Read the model definition and answer for the solid it produces. Units are mm, in the model's axes. Face numbers are marked on the shaded views. A direction names the side the tool comes from. Give positions to 0.01 mm unless a question says otherwise; leave off trailing zeros. Order: outer loops, then holes, each group sorted by start corner. A loop starts at its lowest first (then second) coordinate and runs counter-clockwise, first axis right, second up. Notation, with made-up numbers: (3.5, 81) -> (22.5, 81) arc R22 cw to (22.5, 111) -> close; hole circle Ø6 at (32, 8). An arc over 180 degrees is marked (long way). Use one line per item in the form item = value.
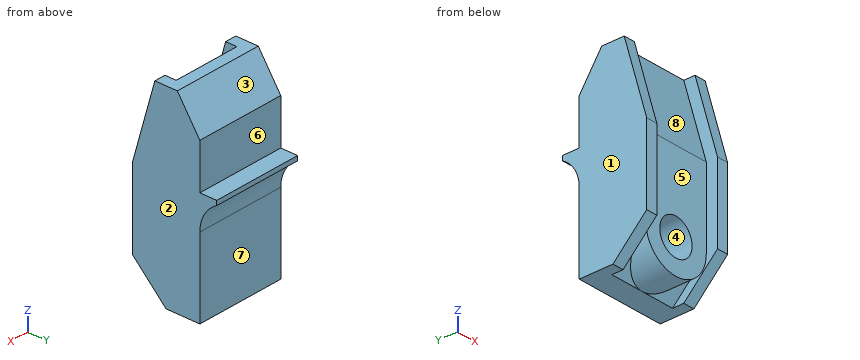
```python
from build123d import *

# Parameters (mm, degrees)
CYLINDER460_R     = 1.6
CYLINDER460_DEPTH = 10
CYLINDER461_R     = 3
CYLINDER461_DEPTH = 3
BOX316_W          = 8
BOX316_H          = 7.5
BOX316_DEPTH      = 17
CHAMFER036_SIZE   = 3
CHAMFER037_SIZE2  = 2
CHAMFER037_SIZE   = 7
BOX317_W          = 6
BOX317_H          = 7.5
BOX317_DEPTH      = 17
BOX314_W          = 10
BOX314_H          = 3
BOX314_DEPTH      = 12
BOX313_W          = 10
BOX313_H          = 3
BOX313_DEPTH      = 12
FILLET112_R       = 2.99
BOX312_W          = 8
BOX312_H          = 7.5
BOX312_DEPTH      = 17
CHAMFER033_SIZE   = 3
CHAMFER034_SIZE2  = 2
CHAMFER034_SIZE   = 7
CHAMFER035_SIZE2  = 3
CHAMFER035_SIZE   = 2


with BuildPart() as cylinder574:
    # Cylinder460 → Cylinder460 (new body)
    with BuildSketch(Plane(origin=(120, -21, 13), x_dir=(1, 0, 0), z_dir=(0, 1, 0))):
        Circle(CYLINDER460_R)
    extrude(amount=CYLINDER460_DEPTH)


with BuildPart() as cylinder575:
    # Cylinder461 → Cylinder461 (new body)
    with BuildSketch(Plane(origin=(120, -15, 13), x_dir=(1, 0, 0), z_dir=(0, 1, 0))):
        Circle(CYLINDER461_R)
    extrude(amount=CYLINDER461_DEPTH)


with BuildPart() as chamfer037:
    # Box316 → Box316 (new body)
    with BuildSketch(Plane(origin=(116, -16, 10), x_dir=(1, 0, 0), z_dir=(0, 0, 1))):
        with Locations((4, 3.75)):
            Rectangle(BOX316_W, BOX316_H)
    extrude(amount=BOX316_DEPTH)

    # Chamfer036
    chamfer036_edges = [chamfer037.edges().sort_by_distance(p)[0] for p in [
        (120, -16, 10),
    ]]
    chamfer(chamfer036_edges, length=CHAMFER036_SIZE)

    # Chamfer037
    chamfer037_edges = [chamfer037.edges().sort_by_distance(p)[0] for p in [
        (120, -16, 27),
    ]]
    chamfer037_side = chamfer037.faces().sort_by_distance((120, -16, 20))[0]
    chamfer(chamfer037_edges, length=CHAMFER037_SIZE, length2=CHAMFER037_SIZE2, reference=chamfer037_side)


with BuildPart() as cut312:
    # Box317 → Box317 (new body)
    with BuildSketch(Plane(origin=(117, -20, 10), x_dir=(1, 0, 0), z_dir=(0, 0, 1))):
        with Locations((3, 3.75)):
            Rectangle(BOX317_W, BOX317_H)
    extrude(amount=BOX317_DEPTH)

    # Cut312: cut Chamfer037
    add(chamfer037.part, mode=Mode.SUBTRACT)


with BuildPart() as cut312_1:
    # Cut312 placement: moved
    add(cut312.part.moved(Location((0, 1, 0))))


with BuildPart() as cube385:
    # Box314 → Box314 (new body)
    with BuildSketch(Plane(origin=(116, -10, 20), x_dir=(1, 0, 0), z_dir=(0, 0, 1))):
        with Locations((5, 1.5)):
            Rectangle(BOX314_W, BOX314_H)
    extrude(amount=BOX314_DEPTH)


with BuildPart() as fillet112:
    # Box313 → Box313 (new body)
    with BuildSketch(Plane(origin=(116, -10, 8), x_dir=(1, 0, 0), z_dir=(0, 0, 1))):
        with Locations((5, 1.5)):
            Rectangle(BOX313_W, BOX313_H)
    extrude(amount=BOX313_DEPTH)

    # Fillet112
    fillet112_edges = [fillet112.edges().sort_by_distance(p)[0] for p in [
        (121, -10, 20),
    ]]
    fillet(fillet112_edges, radius=FILLET112_R)


with BuildPart() as kipper_holder_left:
    # Box312 → Box312 (new body)
    with BuildSketch(Plane(origin=(116, -16, 10), x_dir=(1, 0, 0), z_dir=(0, 0, 1))):
        with Locations((4, 3.75)):
            Rectangle(BOX312_W, BOX312_H)
    extrude(amount=BOX312_DEPTH)

    # Chamfer033
    chamfer033_edges = [kipper_holder_left.edges().sort_by_distance(p)[0] for p in [
        (120, -16, 10),
    ]]
    chamfer(chamfer033_edges, length=CHAMFER033_SIZE)

    # Chamfer034
    chamfer034_edges = [kipper_holder_left.edges().sort_by_distance(p)[0] for p in [
        (120, -16, 27),
    ]]
    chamfer034_side = kipper_holder_left.faces().sort_by_distance((120, -16, 20))[0]
    chamfer(chamfer034_edges, length=CHAMFER034_SIZE, length2=CHAMFER034_SIZE2, reference=chamfer034_side)

    # Cut310: cut Fillet112
    add(fillet112.part, mode=Mode.SUBTRACT)

    # Cut311: cut Cube385
    add(cube385.part, mode=Mode.SUBTRACT)

    # Chamfer035
    chamfer035_edges = [kipper_holder_left.edges().sort_by_distance(p)[0] for p in [
        (120, -10, 27),
    ]]
    chamfer035_side = kipper_holder_left.faces().sort_by_distance((120, -12, 27))[0]
    chamfer(chamfer035_edges, length=CHAMFER035_SIZE, length2=CHAMFER035_SIZE2, reference=chamfer035_side)

    # Cut313: cut Cut312
    add(cut312_1.part, mode=Mode.SUBTRACT)

    # Fusion416: union Cylinder575
    add(cylinder575.part)

    # Cut314: cut Cylinder574
    add(cylinder574.part, mode=Mode.SUBTRACT)


solid = kipper_holder_left.part
```
Item 1: The part is cut by section D-D on y = -10.5. Give the vertices of the cut face in (x, z).
Checks:
outline = (116, 10) -> (124, 10) -> (124, 24.75) -> (116, 24.75) -> close
Item 2: The part is cut by section C-C on x = 121. Give the vertices of the cut face in (y, z).
Checks:
outline = (-15, 10.17) -> (-12.17, 10.17) -> (-12, 10) -> (-10, 10) -> (-10, 17.01) arc R2.99 cw to (-8.5, 19.6) -> (-8.5, 20) -> (-10, 20) -> (-10, 24) -> (-12, 27) -> (-13, 27) -> (-15, 20) -> (-15, 14.25) -> (-11, 14.25) -> (-11, 11.75) -> (-15, 11.75) -> close
Item 3: Given pin 1 Ø1 at (x, z) = (120.5, 13) entering from -Y; pin 2 Ø3 at (x, z) = (121, 12.5) entering from +Y; pin 3 Ø0.8 at (x, y) = (120, -9.5) entering from +Z, each flat-ended and moving along its own axis, determine where each tip first touches the part or whether it passes through.
Checks:
pin_1 = -11
pin_2 = -10
pin_3 = 20
Item 4: Which of the six approach directions +Z, -Z, +X, -X, +Y, -Y give full straight-line access (tool end or side, diameter ignored) to the marked faces 5, 6, 7 and 8?
Checks:
face_5 = +Z, -Z, -Y
face_6 = +Z, +X, -X, +Y
face_7 = -Z, +X, -X, +Y
face_8 = +Z, -Y
Item 5: The part is cut by section A-A on z = 19. Give the vertices of the cut face in (x, y).
Checks:
outline = (116, -16) -> (117, -16) -> (117, -15) -> (123, -15) -> (123, -16) -> (124, -16) -> (124, -9.24) -> (116, -9.24) -> close
Item 6: Determine the mould class of the marked faces 1, 2, 3 and 4 for opening direction X: +X half, -X half, draft (parallel to the pull), parting line (faces both ways), or undercut.
Checks:
face_1 = -X half
face_2 = +X half
face_3 = draft
face_4 = undercut
Item 7: Straight lines are drawn through the part: L1, parallel to X at y = -13.45, z = 13; L2, parallel to X at y = -15.25, z = 21.5; L3, parallel to Z at x = 120, y = -12.45. For each, find the intervals that lie inside material, in ascending order. Write a range as from..to.
Checks:
L1 = 116..118.4, 121.6..124
L2 = 116..117, 123..124
L3 = 10..11.4, 14.6..27
Item 8: The part is cut by section B-B on y = -14.75. Give the vertices of the cut face in (x, z) (3 decimals).
Checks:
outline = (116, 11.75) -> (117, 11.75) -> (117, 12.75) -> (117.01, 12.75) arc R3 ccw to (122.99, 12.75) -> (123, 12.75) -> (123, 11.75) -> (124, 11.75) -> (124, 24.375) -> (123, 24.375) -> (123, 20.875) -> (117, 20.875) -> (117, 24.375) -> (116, 24.375) -> close; hole circle Ø3.2 at (120, 13)
